Source: three-view drawing plus pictorial views. Frame: mm from the lowest corner of the part. A direction names the side the tool comes from. Give positions to 0.01 mm unless a question says otherwise; leave off trailing zeros. Loops run counter-clockwise (first coordinate to the right, second up) from the corner with the lowest first, then second, coordinate; pieces in that order, holes last. Notation, with made-up numbers: (50, 10.25) - (104, 10.25) arc R26 cw to (104, 27.25) - close; hole circle Ø11 at (40, -22.75). An arc over 180 degrees is marked (long way). Answer as a JSON object with one key per item and string values.
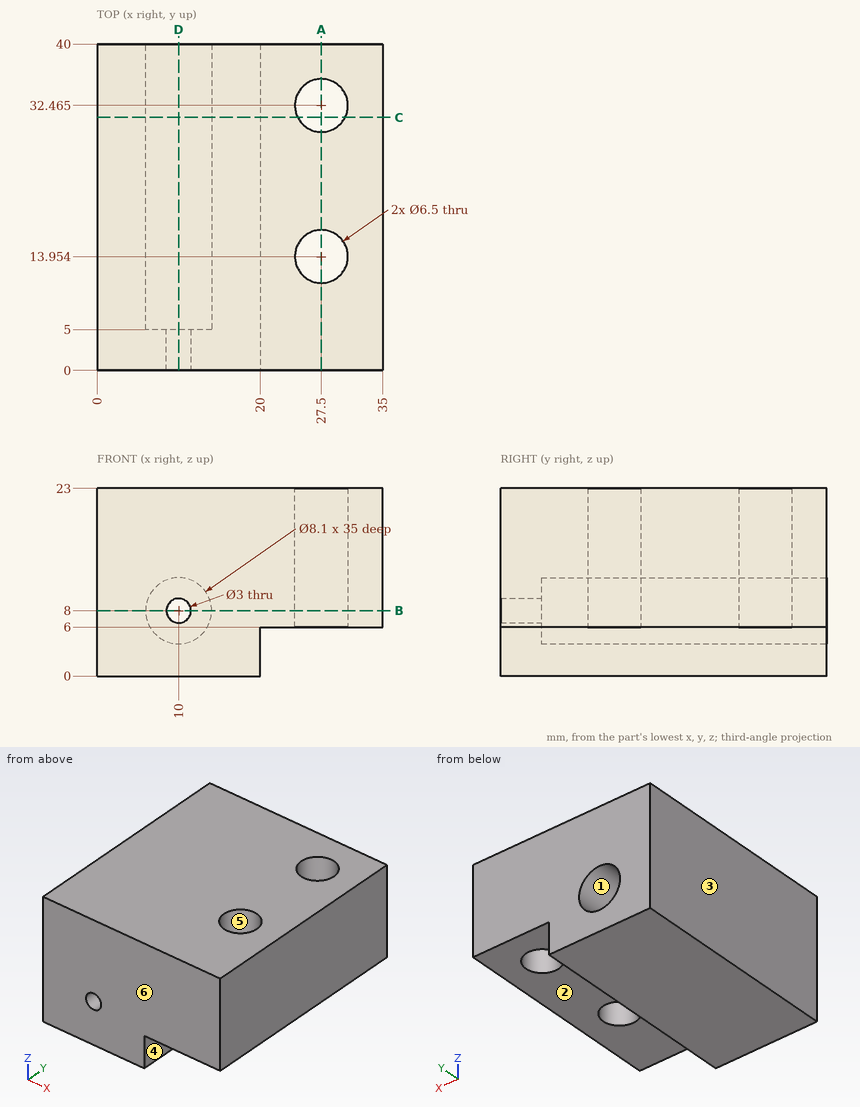
Item 1: Cut plane D-D (x = 10). Return loops of the section in (y, z).
Geometry check:
{"outline": "(0, 0) - (40, 0) - (40, 3.95) - (5, 3.95) - (5, 6.5) - (0, 6.5) - close; (0, 9.5) - (5, 9.5) - (5, 12.05) - (40, 12.05) - (40, 23) - (0, 23) - close"}
Item 2: Material intervals for line 1 (Y direction, x = 27.5, z = 15) (1 decimal); line 2 (Z direction, x = 10, y = 12.5); line 3 (Z direction, x = 33, y = 24), sorted ascending. Write a range as [from, to].
Geometry check:
{"line 1": "y = [0, 10.7], [17.2, 29.2], [35.7, 40]", "line 2": "z = [0, 3.95], [12.05, 23]", "line 3": "z = [6, 23]"}
Item 3: Contact query for flat-ended pins moving along their axis: P1, Ø2.5, axis at x = 8.5, z = 8.5, coming from the +Y side; P2, Ø10.5, axis at x = 27.5, y = 13.95, coming from the -Z side; P3, Ø6, axis at x = 27.5, y = 32.46, coming from the +Z side. Output: stop coordinate, or through.
Geometry check:
{"P1": "stops at y = 5", "P2": "stops at z = 6", "P3": "passes through"}
Item 4: Cut plane C-C (y = 31). Return loops of the section in (x, z).
Geometry check:
{"outline": "(0, 0) - (20, 0) - (20, 6) - (24.6, 6) - (24.6, 23) - (0, 23) - close; (30.4, 6) - (35, 6) - (35, 23) - (30.4, 23) - close; hole circle Ø8.1 at (10, 8)"}
Item 5: Cut plane A-A (x = 27.5). Return loops of the section in (y, z) (1 decimal).
Geometry check:
{"outline": "(0, 6) - (10.7, 6) - (10.7, 23) - (0, 23) - close; (17.2, 6) - (29.2, 6) - (29.2, 23) - (17.2, 23) - close; (35.7, 6) - (40, 6) - (40, 23) - (35.7, 23) - close"}
Item 6: Mould query, pull axis Y, two halves, no side actions, for the marked faces 4, 5 and 6. Classes: released by +Y, released by -Y, zero draft, split by the parting line, or undercut.
Geometry check:
{"face 4": "zero draft", "face 5": "undercut", "face 6": "released by -Y"}
Item 7: Access query for the marked faces 1, 2 and 3. Directions: +Z, -Z, +X, -X, +Y, -Y. A direction counts if a zero-diameter tool reaches every point of the face in a straight line with its end or side. Return the directions, or none.
Geometry check:
{"face 1": "+Y", "face 2": "-Z, +X, +Y, -Y", "face 3": "+Z, -Z, -X, +Y, -Y"}
Item 8: Cut plane B-B (z = 8). Give the number of separate pieces and of enclosed holes in the cut face, then the cut area to 4 significant figures.
Geometry check:
{"separate pieces": "2", "enclosed holes": "2", "area": "1,035 mm2"}
